Could you check a few things on this model? Use its own coordinates, in mm. A direction names the side the tool comes from. Round coordinates to 2 decimals unless told otherwise and drop trailing zeros. Loops run counter-clockwise (first coordinate to the right, second up) from the corner with the lowest first, then second, coordinate; pieces in that order, holes last. Notation, with made-up numbers: (49, -19.75) - (108, -19.75) arc R31 ccw to (108, 11.25) - close; hole circle Ø4 at (-17.5, 72). An arc over 180 degrees is marked (long way). Use one line per item in the form item = value.
```python
from build123d import *

# Parameters (mm, degrees)
SKETCH_1_R          = 7
SKETCH_1_R_2        = 1.6
EXTRUDE_1_DEPTH     = 5
SKETCH_2_R          = 7
EXTRUDE_2_DEPTH     = 2
FILLET_1_R          = 1
CUT_EXTRUDE_1_DEPTH = 1


with BuildPart() as part:
    # 草图1 → 凸台-拉伸1 (new body)
    with BuildSketch(Plane.XY):
        Circle(SKETCH_1_R)
        Circle(SKETCH_1_R_2, mode=Mode.SUBTRACT)
    extrude(amount=EXTRUDE_1_DEPTH)

    # 草图2 → 凸台-拉伸2 (add)
    with BuildSketch(Plane.XY.offset(5)):
        Circle(SKETCH_2_R)
    extrude(amount=EXTRUDE_2_DEPTH)

    # 圆角1
    fillet_1_edges = [part.edges().sort_by_distance(p)[0] for p in [
        (-7, 0, 7),
    ]]
    fillet(fillet_1_edges, radius=FILLET_1_R)

    # 草图4 → 切除-拉伸1 (cut)
    with BuildSketch(Plane.XY.offset(7)):
        Polygon((0, 4.472906985), (-4.833165044, -0.360258059), (-1.762054267, -0.360258059), (-1.762054267, -4.458639339), (1.762054267, -4.458639339), (1.762054267, -0.360258059), (4.833165044, -0.360258059), align=None)
    extrude(amount=-CUT_EXTRUDE_1_DEPTH, mode=Mode.SUBTRACT)


solid = part.part
```
1. If we section it at C-C, the plane z = 3.5: Write out the boundary of the cut face in (x, y).
Solution:
outline = circle Ø14 at (0, 0); hole circle Ø3.2 at (0, 0)
2. On a 3-axis mill with a long thin cutter (end or side, diameter ignored), from which of +Z, -Z, +X, -X, +Y, -Y can I reach the whole of each face in a straight line? I mean faces 5 (the face through (0, 2, 0)), 6 (the face through (2.45, 2.022, 6.507)). Say none if no direction works.
Solution:
face_5 = -Z, +X, -X, +Y, -Y
face_6 = +Z
3. Please list where these lines run through material, in increasing order: line 1 along Y through (x, z) = (0, 2.6); line 2 along Y through (x, z) = (-1.25, 3.75); line 3 along Z through (x, y) = (-2.75, 1.25).
Solution:
line_1 = -7 to -1.6, 1.6 to 7
line_2 = -6.89 to -1, 1 to 6.89
line_3 = 0 to 6
4. For P1, Ø2, axis at x = -4.5, z = 3.5, coming from the +Y side; P2, Ø4, axis at x = 2, y = -2, coming from the -Z side; P3, Ø1, axis at x = 0, y = -1, coming from the -Z side; P4, Ø3, axis at x = 4, z = 5.5, coming from the +Y side, each with a flat end and sliding along its axis, tell me the tip position at first contact or that it passes through.
Solution:
P1 = 6.06
P2 = 0
P3 = 5
P4 = 6.54
5. We'd pull the mould along X, two halves only. Please class faces 1 (the face through (0, 0, 5)), 2 (the face through (3, -1, 7)), 3 (the face through (6.466, -2.681, 2.958)), 4 (the face through (-1.27, -0.97, 2.46)): +X half, -X half, draft (parallel to the pull), parting line (faces both ways), or undercut.
Solution:
face_1 = undercut
face_2 = draft
face_3 = parting line
face_4 = undercut
6. If we section it at A-A, the plane z = 6.25: Write out the boundary of the cut face in (x, y), plus the area to 3 significant figures.
Solution:
outline = circle Ø13.94 at (0, 0); hole (-4.83, -0.36) - (-1.76, -0.36) - (-1.76, -4.46) - (1.76, -4.46) - (1.76, -0.36) - (4.83, -0.36) - (0, 4.47) - close
area = 115 mm^2
7. If we section it at B-B, the plane y = 0: Write out the boundary of the cut face in (x, z).
Solution:
outline = (-7, 0) - (-1.6, 0) - (-1.6, 5) - (1.6, 5) - (1.6, 0) - (7, 0) - (7, 6) arc R1 ccw to (6, 7) - (4.47, 7) - (4.47, 6) - (-4.47, 6) - (-4.47, 7) - (-6, 7) arc R1 ccw to (-7, 6) - close
